from build123d import *

# Parameters (mm, degrees)
F0_R          = 3.6
F1_DEPTH      = 27
F2_COUNT      = 6
F3_R          = 8.75
F4_DEPTH      = 5.6
F4_DEPTH_BACK = 5.6


with BuildPart() as f1:
    # F0 (on Front) → F1 (new body)
    with BuildSketch(Plane.XZ):
        Polygon((-3.233162, -5.6), (3.233162, -5.6), (6.466323, 0), (3.233162, 5.6), (-3.233162, 5.6), (-6.466323, 0), align=None)
        Circle(F0_R, mode=Mode.SUBTRACT)
    extrude(amount=F1_DEPTH)

    # F2: F1 ×6 about axis
    f2_axis = Axis((0, 0, 14.441719), (0, 0, 1))


with BuildPart() as f1_1:
    add(f1.part)
    for i in range(1, F2_COUNT):
        add(f1.part.rotate(f2_axis, i * 360 / F2_COUNT))

    # F3 (on Top) → F4 (join, two sides)
    with BuildSketch(Plane.XY) as f4_sk:
        Circle(F3_R)
    extrude(amount=F4_DEPTH)
    extrude(f4_sk.sketch, amount=-F4_DEPTH_BACK)


solid = f1_1.part
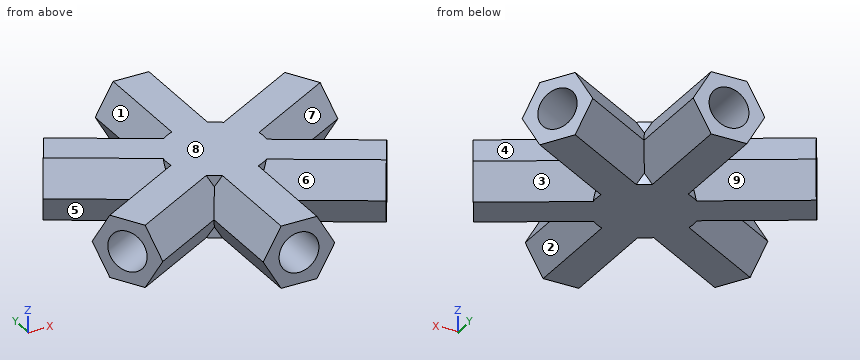
Here's how the part is built. I have some questions about the finished solid (model axes, mm). Face numbers are marked on the shaded views. A direction names the side the tool comes from. Round coordinates to 2 decimals unless told otherwise and drop trailing zeros. Loops run counter-clockwise (first coordinate to the right, second up) from the corner with the lowest first, then second, coordinate; pieces in that order, holes last. Notation, with made-up numbers: M 75,86 L 104,86 A22 cw 104,107 Z; hole C -16,13 d6. An arc over 180 degrees is marked long. Write each question's results on one line, items separated by ' | '. Start each with the question number.
(1) Thinking about a two-plate mould opening in Y: for the marked faces 6, 7, 8 and 9, which applies, pulls with the +Y half, pulls with the -Y half, needs draft (parallel to the pull), parting line crosses it, or undercut?
(2) Will these pins go through, and if not, where does the flat tip stop? P1, Ø5, axis at x = -11.5, z = 0, coming from the +Y side; P2, Ø2, axis at x = -15, z = -1.5, coming from the +Y side; P3, Ø5, axis at x = 11, z = -0.5, coming from the -Y side.
(3) On a 3-axis mill with a long thin cutter (end or side, diameter ignored), from which of +Z, -Z, +X, -X, +Y, -Y can I reach the whole of each face in a straight line? I mean the marked faces 1, 2, 3, 4 and 5. Say none if no direction works.
(4) I want a section at A-A (y = -20). Please give me the cut outline in (x, z).
(5) I want a section at C-C (y = -12). State how many separate pieces and enclosed holes the cut face has, then the cut area to 3 significant figures.
(6) If I drill on probe 1 along Y at (x, z) = (-16, 1.25); probe 2 along X at (y, z) = (7, -2.5); probe 3 along Z at (x, y) = (0, 21), over which ranges is the centre line in solid material (lowest first)? Write a range as from..to.
(7) I want a section at B-B (x = 0). Please give me the cut outline in (y, z).
Solved:
1) face 6: pulls with the -Y half | face 7: undercut | face 8: needs draft | face 9: pulls with the +Y half
2) P1: stops at y = 15.55 | P2: stops at y = 16.01 | P3: stops at y = -15.23
3) face 1: +Z, +Y | face 2: -Z, -Y | face 3: -Z, +X | face 4: +Z, +X | face 5: -Z, -X
4) outline: M -6.47,0 L -3.23,-5.6 L 3.23,-5.6 L 6.47,0 L 3.23,5.6 L -3.23,5.6 Z; hole C 0,0 d7.2
5) separate pieces: 3 | enclosed holes: 1 | area: 233 mm²
6) probe 1: y = -15.87..-13.14, -5.34..-2.6, 2.6..5.34, 13.14..15.87 | probe 2: x = -22.17..-17.31, -6.94..6.94, 17.31..22.17 | probe 3: z = -5.6..-3.6, 3.6..5.6
7) outline: M -27,-5.6 L 27,-5.6 L 27,-3.6 L 8.75,-3.6 L 8.75,3.6 L 27,3.6 L 27,5.6 L -27,5.6 L -27,3.6 L -8.75,3.6 L -8.75,-3.6 L -27,-3.6 Z
